Autodesk Inventor part; units mm, degrees
ref_plane "YZ Plane" through (0, 0, 0) normal (1, 0, 0) x (0, 1, 0)
ref_plane "XZ Plane" through (0, 0, 0) normal (0, 1, 0) x (-1, 0, 0)
ref_plane "XY Plane" through (0, 0, 0) normal (0, 0, 1) x (1, 0, 0)
sketch "Sketch2" plane through (0, 0, 0) normal (1, 0, 0) x (0, 1, 0)
  line L0 (0, 0) -> (25.9, 0)
  line L1 (25.9, 0) -> (25.9, -5)
  line L2 (25.9, -5) -> (26.8, -5)
  line L3 (26.8, -5) -> (26.8, 0)
  line L4 (0, 2) -> (25, 2)
  line L5 (0, 0) -> (-25.9, 0)
  line L6 (-25.9, 0) -> (-25.9, -5)
  line L7 (-25.9, -5) -> (-26.8, -5)
  line L8 (-26.8, -5) -> (-26.8, 0)
  line L9 (0, 2) -> (-25, 2)
  line L10 (0, 0) -> (0, 170)
  line L11 (0, 0) -> (0, 200)
  line L12 (25, 2) -> (25, 0)
  line L13 (-25, 2) -> (-25, 0)
  line L14 (0, 0) -> (0, 198.2)
  spline S0 degree 2 poles (26.8, 0) (0, 400) (-26.8, 0) knots 0 0 0 1 1 1
  spline S1 degree 2 poles (25, 0) (0, 396.4) (-25, 0) knots 0 0 0 1 1 1
  line L15 (0, 170) -> (10.3796, 170)
  line L16 (0, 2) -> (-5, 2)
  line L17 (0, 172) -> (0, 2)
  line L18 (0, 172) -> (10.0276, 172)
  line L19 (0, 0) -> (-5, 0)
  line L20 (-5, 0) -> (-5, 170)
  line L21 (-5, 170) -> (0, 170)
  line L22 (0, 170) -> (0, 0)
  line L23 (-5, 2) -> (-13, 2)
  line L24 (-13, 2) -> (-5, 170)
  line L25 (25, 2) -> (26.6657, 2)
  line L26 (-25, 2) -> (-26.6657, 2)
  line L27 (0, -46.4) -> (0, 243.4)
  point P0 (24.8735, 2)
  point P1 (9.0895, 172)
  point P2 (9.43, 170)
  dimension "d51" = 25.9
  dimension "d52" = 5
  dimension "d53" = 0.9
  dimension "d54" = 2
  dimension "d55" = 25.9
  dimension "d56" = 5
  dimension "d57" = 0.9
  dimension "d58" = 170
  dimension "d59" = 200
  dimension "d60" = 25
  dimension "d61" = 25
  dimension "d62" = 198.2
  dimension "d64" = 25
  dimension "d67" = 2
  dimension "d68" = 170
  dimension "d69" = 5
  dimension "d70" = 8
  dimension "d71" = 170
  dimension "d72" = 87.274
revolve "Revolution5" add sketch "Sketch2" angle 360 mid plane about axis through (0, 0, -10) along (0, 0, 1) contours L10 L4 S1 L0 | L12 L25 S0 L3 L2 L1 L0 | S1 L4 L12 | L4 S1 L15 S0 L25 | L11 L18 S1 L15 | S1 L18 S0 L15 | S1 L11 S0 L18
extrude "Extrusion4" cut sketch "Sketch2" along normal mid plane 60 contours L10 L15 S1 L4 | L9 L20 L21 L10 | L4 S1 L15 S0 L25 | L9 L24 L20
properties part number "nose-basepart1"
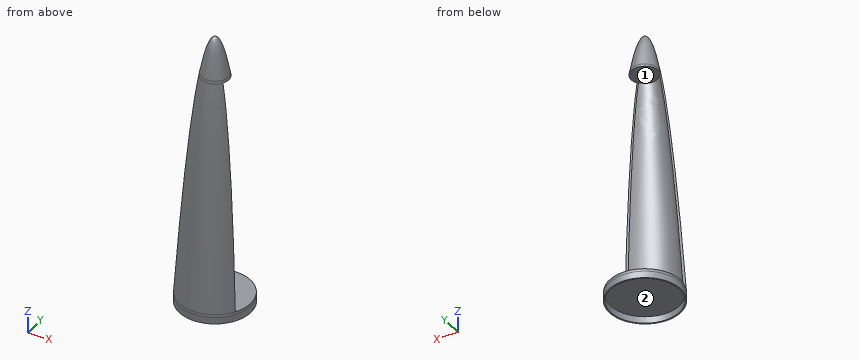
Read the model definition and answer for the solid it produces. Units are mm, in the model's axes. Face numbers are marked on the shaded views. Round coordinates to 2 decimals unless told otherwise and drop trailing zeros.
Q1. Each of these flat-tipped pins is pushed along its axis until it touches: pin 1 (5 mm diameter, centred on x = 12, y = -9, fed in from -Z); pin 2 (5 mm diameter, centred on x = -16.5, z = 107, fed in from +Y); pin 3 (6 mm diameter, centred on x = -10, z = 128, fed in from +Y); pin 4 (4 mm diameter, centred on x = 17, z = 130.5, fed in from -Y). Where does it stop, or does it pass through?
Q2. Section A-A on y = 0 is taken. Give the number of separate pieces and of enclosed holes in the cut face, and give its area (3 significant figures).
Q3. Consider probe 1 along X at (y, z) = (0, -1); probe 2 along Z at (x, y) = (0, -3.5); probe 3 along Z at (x, y) = (16, 3). Determine where each line is inside the solid, lowest interval first.
Q4. Determine the mould class of the marked faces 1 and 2 for opening direction Z: released by +Z, released by -Z, zero draft, split by the parting line, or undercut.
Output:
1. pin 1: stops at z = 0
1. pin 2: stops at y = -7.88
1. pin 3: stops at y = -7.2
1. pin 4: passes through
2. separate pieces: 2
2. enclosed holes: 1
2. area: 214 mm2
3. probe 1: x = -26.8 to -25.9, 25.9 to 26.8
3. probe 2: z = 0 to 2, 170 to 172, 194.32 to 196.59
3. probe 3: z = 0 to 2
4. face 1: undercut
4. face 2: released by -Z
